Can you work these out from the model? Positions are in its coordinate system, mm. Face numbers are marked on the shaded views. Round coordinates to 2 decimals unless told otherwise and drop trailing zeros. Write each loop counter-clockwise with the first axis right and the second up, starting at its lowest first coordinate (ties: lowest second). Pieces come first, ordered by that corner, then holes. Notation, with made-up numbers: (84, -28) - (97, -28) arc R15 cw to (97, -15) - close; hole circle Ø11 at (-12.75, 11.5). An arc over 180 degrees is marked (long way). One line per item, written item: value. Start each with the question number.
(1) Thinking about a two-plate mould opening in X: for the marked faces 1, 2 and 3, which applies, +X half, -X half, draft (parallel to the pull), parting line (faces both ways), or undercut?
(2) If I drill on L1, parallel to Y at x = 149, z = 95; L2, parallel to Z at x = -164.5, y = 30; L3, parallel to Y at x = 168, z = 84.5, over which ranges is the centre line in solid material (lowest first)? Write a range as from..to.
(3) I'm going to push flat-ended pins straight in: pin 1 Ø3.5 at (x, z) = (-124, 145) entering from +Y; pin 2 Ø4 at (y, z) = (51.5, 94.5) entering from -X; pin 3 Ø4.5 at (x, z) = (-189.78, 8.73) entering from +Y; pin 4 Ø6 at (y, z) = (54, 36.5) entering from -X. Where does each tip first touch, or does it pass through?
(4) I want a section at A-A on y = 68.5. Give the number of separate pieces and of enclosed holes in the cut face, plus the area to 3 significant figures.
(5) I want a section at C-C on x = 108. List the corners of the cut face in (y, z) for me, plus the area to 3 significant figures.
(6) I want a section at B-B on z = -84. List the corners of the cut face in (x, y) for me, plus the area to 3 significant figures.
from build123d import *

# Parameters (mm, degrees)
SKETCH1_R                              = 200
BOSS_EXTRUDE1_DEPTH                    = 100
SHELL1_T                               = -20
CBORE_FOR_M5_HEX_HEAD_BOLT2_AT_2_COUNT = 2
CBORE_FOR_M5_HEX_HEAD_BOLT2_AT_2_PITCH = 269.81848572
CBORE_FOR_M5_HEX_HEAD_BOLT2_AT_3_COUNT = 2
CBORE_FOR_M5_HEX_HEAD_BOLT2_AT_3_PITCH = 269.928885586
CBORE_FOR_M5_HEX_HEAD_BOLT2_AT_4_COUNT = 2
CBORE_FOR_M5_HEX_HEAD_BOLT2_AT_4_PITCH = 379.981330262
CBORE_FOR_M5_HEX_HEAD_BOLT2_AT_5_COUNT = 2
CBORE_FOR_M5_HEX_HEAD_BOLT2_AT_5_PITCH = 347.169236891
CBORE_FOR_M5_HEX_HEAD_BOLT2_AT_6_COUNT = 2
CBORE_FOR_M5_HEX_HEAD_BOLT2_AT_6_PITCH = 143.784951156
CBORE_FOR_M5_HEX_HEAD_BOLT2_AT_7_COUNT = 2
CBORE_FOR_M5_HEX_HEAD_BOLT2_AT_7_PITCH = 353.620163975
CBORE_FOR_M5_HEX_HEAD_BOLT2_AT_8_COUNT = 2
CBORE_FOR_M5_HEX_HEAD_BOLT2_AT_8_PITCH = 149.23011883
SHELL5_START                           = 1.4
SHELL5_OUTLINE_R                       = 198.6
SHELL5_OUTLINE_R_2                     = 4.15
SHELL5_DEPTH                           = 17.2
SHELL5_START_2                         = 18.6
SHELL5_2_OUTLINE_R                     = 198.6
SHELL5_2_OUTLINE_R_2                   = 181.4
SHELL5_2_OUTLINE_R_3                   = 4.15
SHELL5_2_DEPTH                         = 76.42
SHELL5_START_3                         = 95.02
SHELL5_3_OUTLINE_R                     = 198.6
SHELL5_3_OUTLINE_R_2                   = 7.52
SHELL5_3_OUTLINE_R_3                   = 181.4
SHELL5_3_DEPTH                         = 3.58


# Read off the part's stored shape, not the designer's step: Shell5
with BuildPart() as part:
    # Sketch1 → Boss-Extrude1 (new body)
    with BuildSketch(Plane(origin=(0, 0, 0), x_dir=(1, 0, 0), z_dir=(0, 1, 0))):
        with Locations(Location((0, 0, 0), (0, 0, 270))):
            Circle(SKETCH1_R)
    extrude(amount=BOSS_EXTRUDE1_DEPTH)

    # Shell1
    shell1_openings = [part.faces().sort_by_distance(p)[0] for p in [
        (0, 100, 0),
    ]]
    offset(amount=SHELL1_T, openings=shell1_openings, kind=Kind.INTERSECTION)

    # Sketch8 → CBORE for M5 Hex Head Bolt2 (revolve, cut)
    with BuildSketch(Plane(origin=(-6.967139306, 100, -189.872217478), x_dir=(0, 0, 1), z_dir=(1, 0, 0))):
        Polygon((0, 0), (0, 100), (2.75, 100), (2.75, 3.58), (6.12, 3.58), (6.12, 0.025), (6.145, 0), align=None)
    cbore_for_m5_hex_head_bolt2 = revolve(axis=Axis((-6.967139306, 106.35, -189.872217478), (0, -1, 0)), mode=Mode.SUBTRACT)

    # CBORE for M5 Hex Head Bolt2 at 2: CBORE for M5 Hex Head Bolt2 ×2
    with Locations(*[Vector(0.7297159379092503, 0, 0.6837504295875969) * (i * CBORE_FOR_M5_HEX_HEAD_BOLT2_AT_2_PITCH) for i in range(1, CBORE_FOR_M5_HEX_HEAD_BOLT2_AT_2_COUNT)]):
        add(cbore_for_m5_hex_head_bolt2, mode=Mode.SUBTRACT)

    # CBORE for M5 Hex Head Bolt2 at 3: CBORE for M5 Hex Head Bolt2 ×2
    with Locations(*[Vector(-0.677264437721292, 0, 0.735739683174737) * (i * CBORE_FOR_M5_HEX_HEAD_BOLT2_AT_3_PITCH) for i in range(1, CBORE_FOR_M5_HEX_HEAD_BOLT2_AT_3_COUNT)]):
        add(cbore_for_m5_hex_head_bolt2, mode=Mode.SUBTRACT)

    # CBORE for M5 Hex Head Bolt2 at 4: CBORE for M5 Hex Head Bolt2 ×2
    with Locations(*[Vector(0.04657327234646247, 0, 0.9989148764048628) * (i * CBORE_FOR_M5_HEX_HEAD_BOLT2_AT_4_PITCH) for i in range(1, CBORE_FOR_M5_HEX_HEAD_BOLT2_AT_4_COUNT)]):
        add(cbore_for_m5_hex_head_bolt2, mode=Mode.SUBTRACT)

    # CBORE for M5 Hex Head Bolt2 at 5: CBORE for M5 Hex Head Bolt2 ×2
    with Locations(*[Vector(0.43983440280673813, 0, 0.8980788930309186) * (i * CBORE_FOR_M5_HEX_HEAD_BOLT2_AT_5_PITCH) for i in range(1, CBORE_FOR_M5_HEX_HEAD_BOLT2_AT_5_COUNT)]):
        add(cbore_for_m5_hex_head_bolt2, mode=Mode.SUBTRACT)

    # CBORE for M5 Hex Head Bolt2 at 6: CBORE for M5 Hex Head Bolt2 ×2
    with Locations(*[Vector(0.9389021515469056, 0, 0.344184180084721) * (i * CBORE_FOR_M5_HEX_HEAD_BOLT2_AT_6_PITCH) for i in range(1, CBORE_FOR_M5_HEX_HEAD_BOLT2_AT_6_COUNT)]):
        add(cbore_for_m5_hex_head_bolt2, mode=Mode.SUBTRACT)

    # CBORE for M5 Hex Head Bolt2 at 7: CBORE for M5 Hex Head Bolt2 ×2
    with Locations(*[Vector(-0.33172041068151087, 0, 0.943377744669276) * (i * CBORE_FOR_M5_HEX_HEAD_BOLT2_AT_7_PITCH) for i in range(1, CBORE_FOR_M5_HEX_HEAD_BOLT2_AT_7_COUNT)]):
        add(cbore_for_m5_hex_head_bolt2, mode=Mode.SUBTRACT)

    # CBORE for M5 Hex Head Bolt2 at 8: CBORE for M5 Hex Head Bolt2 ×2
    with Locations(*[Vector(-0.9046431180155808, 0, 0.4261699532194262) * (i * CBORE_FOR_M5_HEX_HEAD_BOLT2_AT_8_PITCH) for i in range(1, CBORE_FOR_M5_HEX_HEAD_BOLT2_AT_8_COUNT)]):
        add(cbore_for_m5_hex_head_bolt2, mode=Mode.SUBTRACT)

    # Shell5 outline → Shell5 (cut)
    with BuildSketch(Plane(origin=(0, 0, 0), x_dir=(1, 0, 0), z_dir=(0, 1, 0)).offset(SHELL5_START)):
        Circle(SHELL5_OUTLINE_R)
        with Locations((-124.270165325, -143.725175283)):
            Circle(SHELL5_OUTLINE_R_2, mode=Mode.SUBTRACT)
        with Locations((-189.780374227, -8.725175283)):
            Circle(SHELL5_OUTLINE_R_2, mode=Mode.SUBTRACT)
        with Locations((10.729834675, -189.696786077)):
            Circle(SHELL5_OUTLINE_R_2, mode=Mode.SUBTRACT)
        with Locations((145.729834675, -121.913146484)):
            Circle(SHELL5_OUTLINE_R_2, mode=Mode.SUBTRACT)
        with Locations((-141.967139306, 126.274824717)):
            Circle(SHELL5_OUTLINE_R_2, mode=Mode.SUBTRACT)
        with Locations((-6.967139306, 189.872217478)):
            Circle(SHELL5_OUTLINE_R_2, mode=Mode.SUBTRACT)
        with Locations((189.923710067, 5.383711956)):
            Circle(SHELL5_OUTLINE_R_2, mode=Mode.SUBTRACT)
        with Locations((128.032860694, 140.383711956)):
            Circle(SHELL5_OUTLINE_R_2, mode=Mode.SUBTRACT)
    extrude(amount=SHELL5_DEPTH, mode=Mode.SUBTRACT)

    # Shell5 2 outline → Shell5 2 (cut)
    with BuildSketch(Plane(origin=(0, 0, 0), x_dir=(1, 0, 0), z_dir=(0, 1, 0)).offset(SHELL5_START_2)):
        Circle(SHELL5_2_OUTLINE_R)
        Circle(SHELL5_2_OUTLINE_R_2, mode=Mode.SUBTRACT)
        with Locations((-124.270165325, -143.725175283)):
            Circle(SHELL5_2_OUTLINE_R_3, mode=Mode.SUBTRACT)
        with Locations((-189.780374227, -8.725175283)):
            Circle(SHELL5_2_OUTLINE_R_3, mode=Mode.SUBTRACT)
        with Locations((10.729834675, -189.696786077)):
            Circle(SHELL5_2_OUTLINE_R_3, mode=Mode.SUBTRACT)
        with Locations((145.729834675, -121.913146484)):
            Circle(SHELL5_2_OUTLINE_R_3, mode=Mode.SUBTRACT)
        with Locations((-141.967139306, 126.274824717)):
            Circle(SHELL5_2_OUTLINE_R_3, mode=Mode.SUBTRACT)
        with Locations((-6.967139306, 189.872217478)):
            Circle(SHELL5_2_OUTLINE_R_3, mode=Mode.SUBTRACT)
        with Locations((189.923710067, 5.383711956)):
            Circle(SHELL5_2_OUTLINE_R_3, mode=Mode.SUBTRACT)
        with Locations((128.032860694, 140.383711956)):
            Circle(SHELL5_2_OUTLINE_R_3, mode=Mode.SUBTRACT)
    extrude(amount=SHELL5_2_DEPTH, mode=Mode.SUBTRACT)

    # Shell5 3 outline → Shell5 3 (cut)
    with BuildSketch(Plane(origin=(0, 0, 0), x_dir=(1, 0, 0), z_dir=(0, 1, 0)).offset(SHELL5_START_3)):
        Circle(SHELL5_3_OUTLINE_R)
        with Locations((-124.270165325, -143.725175283)):
            Circle(SHELL5_3_OUTLINE_R_2, mode=Mode.SUBTRACT)
        with Locations((-189.780374227, -8.725175283)):
            Circle(SHELL5_3_OUTLINE_R_2, mode=Mode.SUBTRACT)
        with Locations((10.729834675, -189.696786077)):
            Circle(SHELL5_3_OUTLINE_R_2, mode=Mode.SUBTRACT)
        with Locations((145.729834675, -121.913146484)):
            Circle(SHELL5_3_OUTLINE_R_2, mode=Mode.SUBTRACT)
        with Locations((-141.967139306, 126.274824717)):
            Circle(SHELL5_3_OUTLINE_R_2, mode=Mode.SUBTRACT)
        with Locations((-6.967139306, 189.872217478)):
            Circle(SHELL5_3_OUTLINE_R_2, mode=Mode.SUBTRACT)
        Circle(SHELL5_3_OUTLINE_R_3, mode=Mode.SUBTRACT)
        with Locations((189.923710067, 5.383711956)):
            Circle(SHELL5_3_OUTLINE_R_2, mode=Mode.SUBTRACT)
        with Locations((128.032860694, 140.383711956)):
            Circle(SHELL5_3_OUTLINE_R_2, mode=Mode.SUBTRACT)
    extrude(amount=SHELL5_3_DEPTH, mode=Mode.SUBTRACT)


solid = part.part
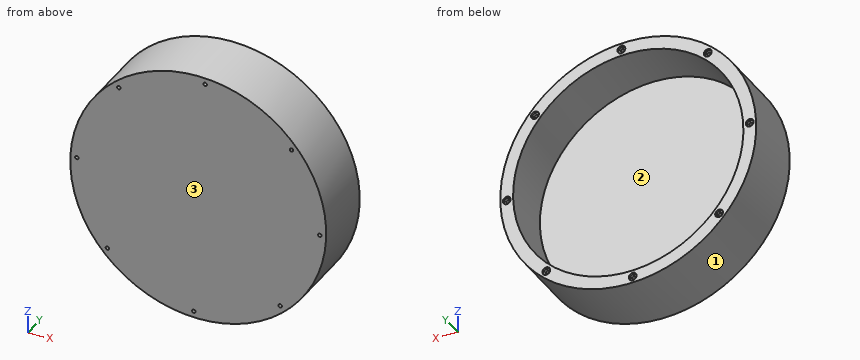
Established:
1. face 1: parting line
1. face 2: undercut
1. face 3: draft
2. L1: 0..1.4, 18.6..20
2. L2: -113.75..-111.27, -76.46..-73.07, 73.07..76.46, 111.27..113.75
2. L3: 0..1.4, 98.6..100
3. pin 1: y = 96.42
3. pin 2: x = -177.32
3. pin 3: through
3. pin 4: x = -197.17
4. separate pieces: 10
4. enclosed holes: 10
4. area: 3,590 mm2
5. outline: (0, -168.33) - (100, -168.33) - (100, -144) - (20, -144) - (20, 144) - (100, 144) - (100, 168.33) - (0, 168.33) - close; hole (1.4, -166.67) - (98.6, -166.67) - (98.6, -145.75) - (18.6, -145.75) - (18.6, 145.75) - (98.6, 145.75) - (98.6, 166.67) - (1.4, 166.67) - close
5. area: 1,550 mm2
6. outline: (-181.5, 0) - (181.5, 0) - (181.5, 100) - (159.2, 100) - (159.2, 20) - (-159.2, 20) - (-159.2, 100) - (-181.5, 100) - close; hole (-179.96, 1.4) - (179.96, 1.4) - (179.96, 98.6) - (160.78, 98.6) - (160.78, 18.6) - (-160.78, 18.6) - (-160.78, 98.6) - (-179.96, 98.6) - close
6. area: 1,570 mm2
